Source: CAD feature listing. Evaluate the final solid. Frame: model axes, mm. Coordinates: 2 decimals unless noted, no trailing zeros. Loops run counter-clockwise (first coordinate to the right, second up) from the corner with the lowest first, then second, coordinate; pieces in that order, holes last. Notation, with made-up numbers: (74, 48) -> (88, 48) arc R12 cw to (88, 61) -> close; hole circle Ø10 at (-20.5, 5). An arc over 180 degrees is marked (long way). Answer as CSV lines item,"result".
from build123d import *

# Parameters (mm, degrees)
BOSS_EXTRUDE1_DEPTH = 7.5
SKETCH3_R           = 2.5
BOSS_EXTRUDE2_DEPTH = 75
SKETCH4_R           = 15
SKETCH4_R_2         = 2.5
CUT_EXTRUDE1_DEPTH  = 528.574777612


with BuildPart() as part:
    # Sketch1 → Boss-Extrude1 (new body)
    with BuildSketch(Plane.XY):
        with BuildLine():
            Line((-34.236900243, -273.477678772), (-14.236900243, -273.477678772))
            Line((-14.236900243, -273.477678772), (34.807854774, -473.477678772))
            ThreePointArc((34.807854774, -473.477678772), (-15.192145226, -523.477678772), (-65.192145226, -473.477678772))
            Line((-65.192145226, -473.477678772), (-34.236900243, -273.477678772))
        make_face()
    extrude(amount=BOSS_EXTRUDE1_DEPTH)

    # Sketch3 → Boss-Extrude2 (add)
    with BuildSketch(Plane(origin=(0, -273.477678772, 0), x_dir=(1, 0, 0), z_dir=(0, 1, 0))):
        with Locations(Location((-24.236900243, -3.75, 0), (0, 0, 270))):
            Circle(SKETCH3_R)
    extrude(amount=BOSS_EXTRUDE2_DEPTH)

    # Sketch4 → Cut-Extrude1 (cut, through all)
    with BuildSketch(Plane.XY.offset(7.5)):
        with Locations((-15.192145226, -473.477678772)):
            Circle(SKETCH4_R)
        with Locations((16.807854774, -473.477678772)):
            Circle(SKETCH4_R_2)
        with Locations((-47.192145226, -473.477678772)):
            Circle(SKETCH4_R_2)
    extrude(amount=-CUT_EXTRUDE1_DEPTH, mode=Mode.SUBTRACT)


solid = part.part
(1) Cut plane D-D (y = -326). Return the cut outline in (x, z), then the cut area to 3 significant figures.
Computed values:
outline,"(-42.37, 0) -> (-1.36, 0) -> (-1.36, 7.5) -> (-42.37, 7.5) -> close"
area,"308 mm^2"
(2) Pin query (flat end, axial travel): pin 1 Ø4 at (x, y) = (16.81, -473.48) entering from -Z; pin 2 Ø4 at (x, z) = (-19, 4) entering from +Y; pin 3 Ø1 at (y, z) = (-467.5, 6.5) entering from +X. Return the tip coordinate at first contact, or that it passes through.
Computed values:
pin 1,"through"
pin 2,"y = -273.48"
pin 3,"x = 33.46"
(3) Cut plane C-C (x = 26.5). Return the cut outline in (y, z).
Computed values:
outline,"(-501.08, 0) -> (-439.6, 0) -> (-439.6, 7.5) -> (-501.08, 7.5) -> close"
(4) Cut plane A-A (z = 3.75). Return the cut outline in (x, y), then the cut area to 3 significant figures.
Computed values:
outline,"(-65.19, -473.48) arc R50 ccw to (34.81, -473.48) -> (-14.24, -273.48) -> (-21.74, -273.48) -> (-21.74, -198.48) -> (-26.74, -198.48) -> (-26.74, -273.48) -> (-34.24, -273.48) -> close; hole circle Ø5 at (-47.19, -473.48); hole circle Ø30 at (-15.19, -473.48); hole circle Ø5 at (16.81, -473.48)"
area,"15,600 mm^2"
(5) Material intervals for L1, parallel to Y at x = -24.5, z = 3.75; L2, parallel to X at y = -467.5, z = 5.25; L3, parallel to Y at x = -25.5, z = 3.25, sorted ascending. Write a range as [from, to].
Computed values:
L1,"[-522.6, -485.24], [-461.71, -198.48]"
L2,"[-64.27, -28.95], [-1.43, 33.34]"
L3,"[-522.4, -484.37], [-462.58, -198.48]"
(6) Draft query along Y for faces 1 (the cylindrical face through (-18.44, -488.12, 3.8)), 2 (the flat face through (-49.93, -374.88, 3.7)), 3 (the cylindrical face through (-14.093, -523.466, 3.698)), 4 (the flat face through (-14, -425, 0)). Return one class per face: released by +Y, released by -Y, zero draft, split by the parting line, or undercut.
Computed values:
face 1,"undercut"
face 2,"released by +Y"
face 3,"released by -Y"
face 4,"zero draft"
(7) Cut plane B-B (y = -260.5). Return the cut outline in (x, z).
Computed values:
outline,"circle Ø5 at (-24.24, 3.75)"
